from build123d import *

# Parameters (mm, degrees)
SKETCH_1_W      = 50
SKETCH_1_H      = 30
EXTRUDE_1_DEPTH = 2
SKETCH_2_W      = 29.42
SKETCH_2_H      = 14.7
EXTRUDE_2_DEPTH = 4
SKETCH_3_W      = 24
SKETCH_3_H      = 15
EXTRUDE_3_DEPTH = 1
SKETCH_4_W      = 16
SKETCH_4_H      = 13
EXTRUDE_4_DEPTH = 2
SKETCH_5_R      = 2.5
EXTRUDE_5_DEPTH = 4


with BuildPart() as part:
    # 草图1 → 凸台-拉伸1 (new body)
    with BuildSketch(Plane(origin=(0, 0, 0), x_dir=(1, 0, 0), z_dir=(0, 1, 0))):
        Rectangle(SKETCH_1_W, SKETCH_1_H)
    extrude(amount=EXTRUDE_1_DEPTH)

    # 草图2 → 凸台-拉伸2 (add)
    with BuildSketch(Plane(origin=(0, 2, 0), x_dir=(1, 0, 0), z_dir=(0, 1, 0))):
        with Locations((5.29, 0)):
            Rectangle(SKETCH_2_W, SKETCH_2_H)
    extrude(amount=EXTRUDE_2_DEPTH)

    # 草图3 → 凸台-拉伸3 (add)
    with BuildSketch(Plane(origin=(0, 0, 0), x_dir=(-1, 0, 0), z_dir=(0, -1, 0))):
        with Locations((-12, 0)):
            Rectangle(SKETCH_3_W, SKETCH_3_H)
    extrude(amount=EXTRUDE_3_DEPTH)

    # 草图4 → 凸台-拉伸4 (add)
    with BuildSketch(Plane.XZ.offset(1)):
        with Locations((9, 0)):
            Rectangle(SKETCH_4_W, SKETCH_4_H)
    extrude(amount=EXTRUDE_4_DEPTH)

    # 草图5 → 凸台-拉伸5 (add)
    with BuildSketch(Plane(origin=(0, 2, 0), x_dir=(1, 0, 0), z_dir=(0, 1, 0))):
        with Locations((-22, 5)):
            Circle(SKETCH_5_R)
        with Locations((-22, -5)):
            Circle(SKETCH_5_R)
        with Locations((-13, -5)):
            Circle(SKETCH_5_R)
        with Locations((-13, 5)):
            Circle(SKETCH_5_R)
        with Locations((-17.5, 0)):
            Circle(SKETCH_5_R)
    extrude(amount=EXTRUDE_5_DEPTH)


solid = part.part
Here's how the part is built. I have some questions about the finished solid (model axes, mm). A direction names the side the tool comes from. Give positions to 0.01 mm unless a question says otherwise; leave off trailing zeros. Order: outer loops, then holes, each group sorted by start corner. A loop starts at its lowest first (then second) coordinate and runs counter-clockwise, first axis right, second up. Notation, with made-up numbers: M 27,-21 L 40,-21 A8 ccw 40,-6 Z; hole C -32.5,38.25 d8. An arc over 180 degrees is marked long. Answer as a JSON object with one key per item and string values. Group by question number.
1) Suppose I cut it at C-C, the plane z = 0. Write out the boundary of the cut face in (x, y), plus the area to 3 significant figures.
2) Suppose I cut it at B-B, the plane y = 3. Write out the boundary of the cut face in (x, z), plus the area to 3 significant figures.
3) Suppose I cut it at D-D, the plane z = -3. Write out the boundary of the cut face in (x, y).
4) On a 3-axis mill with a long thin cutter (end or side, diameter ignored), from which of +Z, -Z, +X, -X, +Y, -Y can I reach the whole of each face in a straight line? I mean faces 4 (the flat face through (5, 4, 7.35)), 5 (the flat face through (5, 4, -7.35)), 6 (the flat face through (12.2, -0.5, 7.5)), 7 (the cylindrical face through (-15.5, 4, -5.1)), 8 (the flat face through (20, 4, 0)). Say none if no direction works.
5) We'd pull the mould along X, two halves only. Please class faces 1 (the flat face through (0, -0.5, 0.1)), 2 (the flat face through (-13, 6, 5)), 3 (the cylindrical face through (-15.5, 4, 4.9)): pulls with the +X half, pulls with the -X half, needs draft (parallel to the pull), parting line crosses it, or undercut.
6) Suppose I cut it at A-A, the plane x = -17.5. Write out the boundary of the cut face in (y, z), plus the area to 3 significant figures.
7) I'm going to push flat-ended pins straight in: pin 1 Ø1.6 at (y, z) = (-2, 2.5) entering from -X; pin 2 Ø4.5 at (x, y) = (9, 4.5) entering from -Z; pin 3 Ø2 at (x, z) = (-17.5, 0.5) entering from -Y. Where does each tip first touch, or does it pass through?
8) Please list where these lines run through material, in increasing order: L1, parallel to X at y = 2.25, z = -4; L2, parallel to Z at x = -3.5, y = 3.5; L3, parallel to Y at x = -10, z = -11.5. Write a range as [from, to].
Results found:
{
 "1": {"outline": "M -25,0 L 0,0 L 0,-1 L 1,-1 L 1,-3 L 17,-3 L 17,-1 L 24,-1 L 24,0 L 25,0 L 25,2 L 20,2 L 20,6 L -9.42,6 L -9.42,2 L -15,2 L -15,6 L -20,6 L -20,2 L -25,2 Z", "area": "294 mm²"},
 "2": {"outline": "C -22,-5 d5; C -22,5 d5; C -17.5,0 d5; C -13,-5 d5; C -13,5 d5; M -9.42,-7.35 L 20,-7.35 L 20,7.35 L -9.42,7.35 Z", "area": "531 mm²"},
 "3": {"outline": "M -25,0 L 0,0 L 0,-1 L 1,-1 L 1,-3 L 17,-3 L 17,-1 L 24,-1 L 24,0 L 25,0 L 25,2 L 20,2 L 20,6 L -9.42,6 L -9.42,2 L -11.5,2 L -11.5,6 L -14.5,6 L -14.5,2 L -20.5,2 L -20.5,6 L -23.5,6 L -23.5,2 L -25,2 Z"},
 "4": {"face 4": "+Z, +X, +Y", "face 5": "-Z, +X, +Y", "face 6": "+Z, +X, -X, -Y", "face 7": "+Y", "face 8": "+Z, -Z, +X, +Y"},
 "5": {"face 1": "pulls with the -X half", "face 2": "needs draft", "face 3": "undercut"},
 "6": {"outline": "M 0,-15 L 2,-15 L 2,-2.5 L 6,-2.5 L 6,2.5 L 2,2.5 L 2,15 L 0,15 Z", "area": "80.0 mm²"},
 "7": {"pin 1": "x = 1", "pin 2": "z = -7.35", "pin 3": "y = 0"},
 "8": {"L1": "[-24.29, -19.71], [-15.29, -10.71], [-9.42, 20]", "L2": "[-7.35, 7.35]", "L3": "[0, 2]"}
}
